Source: CAD feature listing. Evaluate the final solid. Frame: model axes, mm. Face numbers are marked on the shaded views. A direction names the side the tool comes from. Coordinates: 2 decimals unless noted, no trailing zeros. Order: outer loops, then holes, each group sorted by start corner. A loop starts at its lowest first (then second) coordinate and runs counter-clockwise, first axis right, second up. Notation, with made-up numbers: (-24.75, 57.5) - (-19.75, 57.5) arc R13 cw to (-19.75, 82.5) - close; hole circle Ø10 at (20, 27.5). An arc over 180 degrees is marked (long way). One line per question, with ' | ' between items. Start each with the question number.
(1) Section B-B (y = 12.5). Return the cut outline in (x, z), then the cut area to 3 significant figures.
(2) Section D-D (z = 15). Return the cut outline in (x, y), then the cut area to 3 significant figures.
(3) Access query for the marked faces 1, 2, 3, 4 and 5. Directions: +Z, -Z, +X, -X, +Y, -Y. A direction counts if a zero-diameter tool reaches every point of the face in a straight line with its end or side. Return the directions, or none.
(4) Section A-A (z = -5). Return the cut outline in (x, y), then the cut area to 3 significant figures.
(5) Draft query along Z for the marked faces 6, 7 and 8. Return one class per face: +Z half, -Z half, draft (parallel to the pull), parting line (faces both ways), or undercut.
(6) Line query: line 1 along Y through (x, z) = (0, 4.5); line 2 along X through (y, z) = (0, 8.25); line 3 along X through (y, z) = (-8.5, 17.5). Output: solid intervals per line, ascending.
(7) Contact query for flat-ended pins moving along their axis: P1, Ø6, axis at y = -11.5, z = 15, coming from the +X side; P2, Ø15.5, axis at x = 0, y = 0, coming from the +Z side; P3, Ø4, axis at x = 0, y = 1.5, coming from the -Z side; P4, Ø3, axis at y = -11.5, z = -5, coming from the +X side. Output: stop coordinate, or through.
from build123d import *

# Parameters (mm, degrees)
EXTRUDE_1_DEPTH      = 10
SKETCH_10_W          = 40
SKETCH_10_H          = 34
EXTRUDE_3_DEPTH      = 5
SKETCH_11_R          = 2.6
CUT_EXTRUDE_7_DEPTH  = 40.230090492
SKETCH_2_R           = 11.1
CUT_EXTRUDE_1_DEPTH  = 7
SKETCH_3_R           = 6
CUT_EXTRUDE_2_DEPTH  = 1
SKETCH_14_R          = 11.5
CUT_EXTRUDE_10_DEPTH = 35.684290392
CHAMFER_1_SIZE       = 0.4
FILLET_1_R           = 2.5


with BuildPart() as part:
    # Эскиз1 → Бобышка-Вытянуть1 (new body)
    with BuildSketch(Plane.XY):
        with BuildLine():
            Line((0, 17), (-13, 17))
            Line((-13, 17), (-13, -17))
            Line((-13, -17), (0, -17))
            ThreePointArc((0, -17), (17, 0), (0, 17))
        make_face()
    extrude(amount=EXTRUDE_1_DEPTH)

    # Эскиз10 → Бобышка-Вытянуть3 (add)
    with BuildSketch(Plane.ZY.offset(13)):
        with Locations((5, 0)):
            Rectangle(SKETCH_10_W, SKETCH_10_H)
    extrude(amount=-EXTRUDE_3_DEPTH)

    # Эскиз11 → Вырез-Вытянуть7 (cut, through all)
    with BuildSketch(Plane(origin=(-8, 0, 0), x_dir=(0, 0, -1), z_dir=(1, 0, 0))):
        with Locations(Location((5, -11.5, 0), (0, 0, 90))):
            Circle(SKETCH_11_R)
        with Locations(Location((5, 11.5, 0), (0, 0, 90))):
            Circle(SKETCH_11_R)
        with Locations(Location((-15, 11.5, 0), (0, 0, 90))):
            Circle(SKETCH_11_R)
        with Locations(Location((-15, -11.5, 0), (0, 0, 90))):
            Circle(SKETCH_11_R)
    extrude(amount=-CUT_EXTRUDE_7_DEPTH, mode=Mode.SUBTRACT)

    # Эскиз2 → Вырез-Вытянуть1 (cut)
    with BuildSketch(Plane.XY.offset(10)):
        Circle(SKETCH_2_R)
    extrude(amount=-CUT_EXTRUDE_1_DEPTH, mode=Mode.SUBTRACT)

    # Эскиз3 → Вырез-Вытянуть2 (cut)
    with BuildSketch(Plane.XY.offset(3)):
        Circle(SKETCH_3_R)
    extrude(amount=-CUT_EXTRUDE_2_DEPTH, mode=Mode.SUBTRACT)

    # Эскиз14 → Вырез-Вытянуть10 (cut, through all)
    with BuildSketch(Plane.XY.offset(10)):
        Circle(SKETCH_14_R)
    extrude(amount=CUT_EXTRUDE_10_DEPTH, mode=Mode.SUBTRACT)

    # Фаска1
    chamfer_1_edges = [part.edges().sort_by_distance(p)[0] for p in [
        (-11.1, 0, 10),
    ]]
    chamfer(chamfer_1_edges, length=CHAMFER_1_SIZE - 0.0001)  # a hair under: the kernel refuses the full size

    # Скругление1
    fillet_1_edges = [part.edges().sort_by_distance(p)[0] for p in [
        (-10.5, 17, -15),
        (-10.5, 17, 25),
        (-10.5, -17, 25),
        (-10.5, -17, -15),
    ]]
    fillet(fillet_1_edges, radius=FILLET_1_R)


solid = part.part
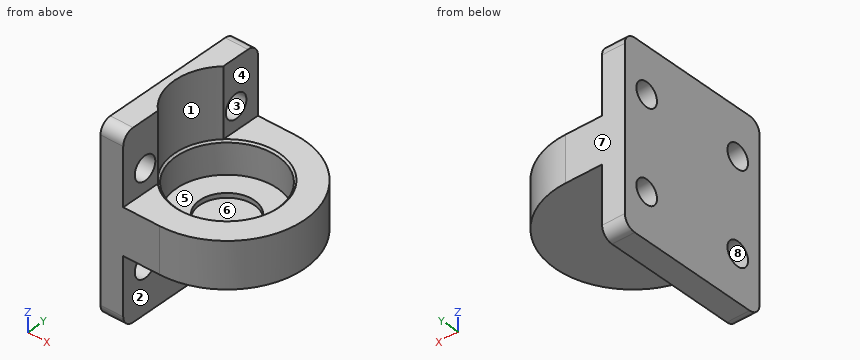
Response values:
1) outline: (-13, -15) - (-8, -15) - (-8, -7.4) - (-13, -7.4) - close; (-13, -2.6) - (-8, -2.6) - (-8, 0) - (11.52, 0) - (11.52, 10) - (-8, 10) - (-8, 12.6) - (-13, 12.6) - close; (-13, 17.4) - (-8, 17.4) - (-8, 25) - (-13, 25) - close | area: 347 mm²
2) outline: (-13, -17) - (-8, -17) - (-8, -14.1) - (-13, -14.1) - close; (-13, -8.9) - (-8, -8.9) - (-8, -8.26) arc R11.5 cw to (-8, 8.26) - (-8, 8.9) - (-13, 8.9) - close; (-13, 14.1) - (-8, 14.1) - (-8, 17) - (-13, 17) - close | area: 78.1 mm²
3) face 1: +Z, +X | face 2: -Z, +X, +Y, -Y | face 3: +X, -X | face 4: +Z, +X, +Y, -Y | face 5: +Z
4) outline: (-13, -17) - (-8, -17) - (-8, -14.1) - (-13, -14.1) - close; (-13, -8.9) - (-8, -8.9) - (-8, 8.9) - (-13, 8.9) - close; (-13, 14.1) - (-8, 14.1) - (-8, 17) - (-13, 17) - close | area: 118 mm²
5) face 6: +Z half | face 7: draft | face 8: undercut
6) line 1: y = -17 to -11.1, 11.1 to 17 | line 2: x = -13 to -11.1, 11.1 to 17 | line 3: x = -13 to -8
7) P1: stops at x = -8 | P2: stops at z = 3 | P3: stops at z = 0 | P4: passes through
